from build123d import *

# Parameters (mm, degrees)
CHAMFER_1_SIZE           = 0.4
PATTERN_CIRCULAR_1_COUNT = 3


with BuildPart() as part:
    # Эскиз1 → Повернуть1 (revolve)
    with BuildSketch(Plane(origin=(0, 0, 0), x_dir=(0, 0, -1), z_dir=(1, 0, 0)), mode=Mode.PRIVATE) as revolve_1_sk:
        Polygon((0, 0), (0, -1.5), (9.4, -1.5), (9.4, -5), (10.4, -5), (10.4, -8), (66.4, -8), (66.4, 0), align=None)
    revolve(revolve_1_sk.sketch.rotate(Axis((0, 0, 0), (0, 0, -1)), 270), axis=Axis((0, 0, 0), (0, 0, -1)))

    # Фаска1
    chamfer_1_edges = [part.edges().sort_by_distance(p)[0] for p in [
        (-1.5, 0, 0),
    ]]
    chamfer(chamfer_1_edges, length=CHAMFER_1_SIZE)

    # Эскиз5 → Отверстие обработанное метчиком M2x0.41 (revolve, cut)
    with BuildSketch(Plane(origin=(0, 6.5, -10.4), x_dir=(0, -1, 0), z_dir=(1, 0, 0))):
        Polygon((0, 0), (0, 4.480688495), (0.8, 4), (0.8, 0.225), (1.025, 0), align=None)
    m2x0_41 = revolve(axis=Axis((0, 6.5, -4.05), (0, 0, -1)), mode=Mode.SUBTRACT)

    # Круговой массив1: Отверстие обработанное метчиком M2x0.41 ×3 about axis
    pattern_circular_1_axis = Axis((0, 0, 0), (0, 0, 1))
    for i in range(1, PATTERN_CIRCULAR_1_COUNT):
        add(m2x0_41.rotate(pattern_circular_1_axis, i * 360 / PATTERN_CIRCULAR_1_COUNT), mode=Mode.SUBTRACT)


solid = part.part
Part model, mm, in its own coordinate system. A direction names the side the tool comes from. Give positions to 0.01 mm unless a question says otherwise; leave off trailing zeros. Write each loop counter-clockwise with the first axis right and the second up, starting at its lowest first coordinate (ties: lowest second). Pieces come first, ordered by that corner, then holes.
1) Which spindle directions (+Z, -Z, +X, -X, +Y, -Y) get a long thin tool onto all of the face, cutting with end or side? Do faces 1 (the face through (0, 0, -66.4)), 2 (the face through (-6.422, -3.146, -12.486)). Say none if no direction does.
Resolved:
face 1: -Z, +X, -X, +Y, -Y
face 2: +Z
2) Probe L1, parallel to X at y = -3.25, z = -11.6; L2, parallel to Y at x = 0, z = -11.75; L3, parallel to Z at x = 5.5, y = 1.75. List the from-to ranges inside material, lowest first.
Resolved:
L1: x = -7.31 to -6.43, -4.83 to 4.83, 6.43 to 7.31
L2: y = -8 to 5.7, 7.3 to 8
L3: z = -66.4 to -10.4
3) Cut at A-A on y = 2.25. Write the cut outline in (x, z), then the cut area to 3 significant figures.
Resolved:
outline: (-7.68, -66.4) - (7.68, -66.4) - (7.68, -10.4) - (4.47, -10.4) - (4.47, -9.4) - (-4.47, -9.4) - (-4.47, -10.4) - (-7.68, -10.4) - close
area: 869 mm2
4) Cut at B-B on z = -21. Write the cut outline in (x, y).
Resolved:
outline: circle Ø16 at (0, 0)
5) Pin check, flat tips, straight feed: pin 1 (2 mm diameter, centred on x = -5.5, y = -4, fed in from +Z); pin 2 (1 mm diameter, centred on x = -5.63, y = -3.25, fed in from +Z); pin 3 (6 mm diameter, centred on x = 2, z = -7.5, fed in from +Y). Stop position of each tip, or through.
Resolved:
pin 1: stops at z = -10.4
pin 2: stops at z = -14.58
pin 3: stops at y = 7.9
6) Two-plate mould, pull along Y, no slides. Class faces 3 (the face through (1.43, -0.45, -4.96)), 4 (the face through (0.1, 5.2, -10.4)), 5 (the face through (-5.545, -3.14, -14.797)): released by +Y, released by -Y, zero draft, split by the parting line, or undercut.
Resolved:
face 3: split by the parting line
face 4: zero draft
face 5: undercut
